Work out the finished part from the listing and answer in its coordinate system (mm). Coordinates: 2 decimals unless noted, no trailing zeros. Write each loop counter-clockwise with the first axis right and the second up, starting at its lowest first coordinate (ties: lowest second). Pieces come first, ordered by that corner, then holes. Notation, with made-up numbers: M 71.5,-7.75 L 100.5,-7.75 A26 ccw 100.5,20.25 Z; hole C 55,14.25 d6. An arc over 180 degrees is marked long. Use CSV: the item, a comma, the result in double quotes.
from build123d import *

# Parameters (mm, degrees)
SKETCH1_R           = 9
BOSS_EXTRUDE1_DEPTH = 25
SKETCH2_R           = 3
CUT_EXTRUDE1_DEPTH  = 25
SKETCH3_R           = 4
CUT_EXTRUDE2_DEPTH  = 12.5
CUT_SWEEP1_PITCH    = 1.875


with BuildPart() as part:
    # Sketch1 → Boss-Extrude1 (new body)
    with BuildSketch(Plane.XY):
        Circle(SKETCH1_R)
    extrude(amount=BOSS_EXTRUDE1_DEPTH)

    # Sketch2 → Cut-Extrude1 (cut)
    with BuildSketch(Plane.XY.offset(25)):
        Circle(SKETCH2_R)
    extrude(amount=-CUT_EXTRUDE1_DEPTH, mode=Mode.SUBTRACT)

    # Sketch3 → Cut-Extrude2 (cut)
    with BuildSketch(Plane(origin=(0, 0, 0), x_dir=(-1, 0, 0), z_dir=(0, 0, -1))):
        Circle(SKETCH3_R)
    extrude(amount=-CUT_EXTRUDE2_DEPTH, mode=Mode.SUBTRACT)

    # Cut-Sweep1: the profile of Sketch4 screwed along a right-hand helix of 4 turns, 10 arcs to a turn; built about Z, then put on its axis
    cut_sweep1_z = Axis((0, 0, 0), (0, 0, 1))
    cut_sweep1_corners = [(1.343280354, 0, 0), (1.343280354, 0, 0.25), (9.561008436, 0, 0.25), (9.561008436, 0, 0)]
    with BuildLine(mode=Mode.PRIVATE) as cut_sweep1_profile:
        Line(cut_sweep1_corners[0], cut_sweep1_corners[1])
        Line(cut_sweep1_corners[1], cut_sweep1_corners[2])
        Line(cut_sweep1_corners[2], cut_sweep1_corners[3])
        Line(cut_sweep1_corners[3], cut_sweep1_corners[0])
    cut_sweep1_cap = Face(cut_sweep1_profile.wire())
    cut_sweep1_turn_angles = [0, 18, 36, 54, 72, 90, 108, 126, 144, 162, 180, 198, 216, 234, 252, 270, 288, 306, 324, 342, 360]
    cut_sweep1_turn_weights = [1, 0.9510565162951535, 1, 0.9510565162951535, 1, 0.9510565162951535, 1, 0.9510565162951535, 1, 0.9510565162951535, 1, 0.9510565162951535, 1, 0.9510565162951535, 1, 0.9510565162951535, 1, 0.9510565162951535, 1, 0.9510565162951535, 1]
    cut_sweep1_turn_rails = [Edge.make_bspline([Vector(p[0], p[1], 0).rotate(cut_sweep1_z, cut_sweep1_turn_angles[k]) / cut_sweep1_turn_weights[k] + Vector(0, 0, p[2] + CUT_SWEEP1_PITCH * cut_sweep1_turn_angles[k] / 360) for k in range(21)], [0, 0, 0, 1, 1, 2, 2, 3, 3, 4, 4, 5, 5, 6, 6, 7, 7, 8, 8, 9, 9, 10, 10, 10], 2, cut_sweep1_turn_weights) for p in cut_sweep1_corners]
    cut_sweep1_turn_sides = [Face.make_surface_from_curves(cut_sweep1_turn_rails[p[0]], cut_sweep1_turn_rails[p[1]]) for p in [(0, 1), (1, 2), (2, 3), (3, 0)]]
    cut_sweep1 = Plane(origin=(0, 0, 16.66666667), x_dir=(0, -1, 0), z_dir=(0, 0, -1)) * Solid(Shell([*[p.moved(Location((0, 0, CUT_SWEEP1_PITCH * i))) for i in range(4) for p in cut_sweep1_turn_sides], cut_sweep1_cap, cut_sweep1_cap.rotate(cut_sweep1_z, 1440).moved(Location((0, 0, CUT_SWEEP1_PITCH * 1440 / 360)))]))
    add(cut_sweep1, mode=Mode.SUBTRACT)


solid = part.part
Item 1: Given pin 1 (10.5 mm diameter, centred on x = 0, y = 0, fed in from -Z); pin 2 (3 mm diameter, centred on y = -7, z = 8, fed in from -X); pin 3 (3 mm diameter, centred on y = -2.5, z = 16, fed in from -X); pin 4 (1 mm diameter, centred on x = -5, z = 8.5, fed in from +Y), each flat-ended and moving along its own axis, determine where each tip first touches the part or whether it passes through.
Answer:
pin 1,"stops at z = 0"
pin 2,"stops at x = -7.12"
pin 3,"stops at x = -8.94"
pin 4,"stops at y = 7.79"
Item 2: The part is cut by section B-B (z = 19). Write down the section's boundary in (x, y).
Answer:
outline,"C 0,0 d18; hole C 0,0 d6"
Item 3: The part is cut by section A-A (x = -0.5). Count the separate pieces of the cut face and the enclosed holes in it, then the cut area to 3 significant figures.
Answer:
separate pieces,"10"
enclosed holes,"0"
area,"265 mm2"
Item 4: For a pull along Y with two mould halves and no side action, classify faces 1 (the face through (4, -2, 0)), 2 (the face through (3, 1, 12.5)) as released by +Y, released by -Y, zero draft, split by the parting line, or undercut.
Answer:
face 1,"zero draft"
face 2,"undercut"
Item 5: Consider probe 1 along X at (y, z) = (0, 11.6); probe 2 along X at (y, z) = (0, 20.75); probe 3 along Z at (x, y) = (-4.5, -2.25). Determine where each line is inside the solid, lowest interval first.
Answer:
probe 1,"x = -9 to -4, 4 to 9"
probe 2,"x = -9 to -3, 3 to 9"
probe 3,"z = 0 to 10.46, 10.71 to 12.34, 12.59 to 14.21, 14.46 to 16.09, 16.34 to 25"
